from build123d import *

# Parameters (mm, degrees)
F0_W     = 19.05
F0_H     = 38.1
F1_DEPTH = 127
F2_R     = 18.0975
F3_DEPTH = 19.05
F5_R     = 3.96875
F6_DEPTH = 39.371
F8_DEPTH = 19.051


with BuildPart() as f1:
    # F0 (on Front) → F1 (new body, symmetric)
    with BuildSketch(Plane.XZ):
        with Locations((9.525, 19.05)):
            Rectangle(F0_W, F0_H)
    extrude(amount=F1_DEPTH, both=True)


with BuildPart() as f3:
    # F2 (on face) → F3 (new body)
    with BuildSketch(Plane.YZ.offset(19.05)):
        with BuildLine():
            Line((-127, 10.535887), (-127, 29.469113))
            ThreePointArc((-127, 29.469113), (-167.3225, 20.0025), (-127, 10.535887))
        make_face()
        with Locations((-146.05, 20.0025)):
            Circle(F2_R, mode=Mode.SUBTRACT)
    extrude(amount=-F3_DEPTH)

    # F4: union F1
    add(f1.part)

    # F5 (on face) → F6 (cut, through all)
    with BuildSketch(Plane.XY.offset(38.1)):
        with Locations((9.525, 25.4)):
            Circle(F5_R)
    extrude(amount=-F6_DEPTH, mode=Mode.SUBTRACT)

    # F7 (on face) → F8 (cut, through all)
    with BuildSketch(Plane(origin=(0, 0, 0), x_dir=(0, -1, 0), z_dir=(-1, 0, 0))):
        Polygon((-127, 0), (25.4, 0), (-40.591136, 38.1), (-127, 38.1), align=None)
    extrude(amount=-F8_DEPTH, mode=Mode.SUBTRACT)


solid = f3.part
For this review, take the finished solid that the model builds, in its own axes (mm). A direction names the side the tool comes from. Give positions to 0.01 mm unless a question says otherwise; leave off trailing zeros. Loops run counter-clockwise (first coordinate to the right, second up) from the corner with the lowest first, then second, coordinate; pieces in that order, holes last. Notation, with made-up numbers: M 89.5,-5.5 L 112.5,-5.5 A31 ccw 112.5,29.5 Z; hole C -3,83.25 d8. An arc over 180 degrees is marked long. Answer as a JSON object with one key per item and string values. Group by question number.
Q1. For probe 1 along Y at (x, z) = (14.75, 36.5); probe 2 along Y at (x, z) = (8, 30); probe 3 along X at (y, z) = (25.4, 32.5), list the stretches that pass through material, from the lowest coordinate up. Write a range as [from, to].
Q2. Tool access review of faces 1 (the flat face through (9, -44, 38.1)), 2 (the flat face through (9, -77, 0)), 3 (the flat face through (19.05, -65, 20)): name each direction out of +Z, -Z, +X, -X, +Y, -Y from which nothing blocks a thin tool from reaching the whole face with its end or side.
Q3. Insertion check: P1, Ø1.5, axis at x = 13, y = -109.5, coming from the +Z side; P2, Ø6, axis at x = 3.5, z = 21.5, coming from the -Y side; P3, Ø8, axis at x = 12, z = 35, coming from the -Y side. Each pin has a flat end and moves straight along its axis. Give the tip position at first contact, or say it passes through.
Q4. Mouldability with a two-part tool opening along Y and no side actions: class faces 4 (the flat face through (9.39, 7.13, 18.78)), 5 (the flat face through (0, -65, 20)), 6 (the flat face through (9, -127, 5)) as +Y half, -Y half, draft (parallel to the pull), parting line (faces both ways), or undercut.
Q5. Add section A-A on z = 33.5. Give the number of separate pieces and of enclosed holes in the cut face, and give its area (3 significant figures).
Q6. Add section B-B on y = -146.05. Give the boundary of the cut face in (x, z) (3 decimals).
Checked values:
{
 "1": {"probe 1": "[-159.48, -153.49], [-138.61, -132.62], [-127, 37.82]", "probe 2": "[-164.83, -161.14], [-130.96, -127.27], [-127, 21.74]", "probe 3": "[0, 5.56], [13.49, 19.05]"},
 "2": {"face 1": "+Z, +X, -X, +Y", "face 2": "-Z, +X, -X, +Y", "face 3": "+Z, -Z, +X, +Y, -Y"},
 "3": {"P1": "z = 38.1", "P2": "y = -167.32", "P3": "y = -164.26"},
 "4": {"face 4": "+Y half", "face 5": "draft", "face 6": "undercut"},
 "5": {"separate pieces": "3", "enclosed holes": "1", "area": "3,160 mm²"},
 "6": {"outline": "M 0,-1.27 L 19.05,-1.27 L 19.05,1.905 L 0,1.905 Z; M 0,38.1 L 19.05,38.1 L 19.05,41.275 L 0,41.275 Z"}
}
